Read the model definition and answer for the solid it produces. Units are mm, in the model's axes. A direction names the side the tool comes from. Give positions to 0.01 mm unless a question says otherwise; leave off trailing zeros. Loops run counter-clockwise (first coordinate to the right, second up) from the corner with the lowest first, then second, coordinate; pieces in that order, holes last.
(1) Find section B-B, the plane x = -7.5. Write down the section's boundary in (y, z).
(2) Each of these flat-tipped pins is pushed along its axis until it touches: P1, Ø2, axis at x = -6, z = 5, coming from the -Y side; P2, Ø1.5, axis at x = -4, y = 0, coming from the +Z side; P3, Ø0.6, axis at x = 3.5, z = 5, coming from the +Y side. Where does it stop, or does it pass through?
(3) Determine the mould class of faces 3 (the face through (-16.339, -7.547, 2.958)), 4 (the face through (-2.483, -7.657, 5.246)), 5 (the face through (-2, -8, 5.5)), 6 (the face through (0, 11, 6)) for opening direction X: pulls with the +X half, pulls with the -X half, needs draft (parallel to the pull), parting line crosses it, or undercut.
(4) Straight lines are drawn through the part: probe 1 along X at (y, z) = (-11, 5.25); probe 2 along Z at (x, y) = (-5.5, -5); probe 3 along Z at (x, y) = (4.5, -5.5). For each, find the intervals that lie inside material, in ascending order.
(5) Find section A-A, the plane z = 2.5. Write down the section's boundary in (x, y).
(6) Find section D-D, the plane x = -14. Write down the section's boundary in (y, z), then the cut area to 3 significant figures.
(7) Which of the six approach directions +Z, -Z, +X, -X, +Y, -Y give full straight-line access (tool end or side, diameter ignored) to faces 1 (the face through (0, 6, 0)), 2 (the face through (2.28, -7.66, 5.25))?
(8) Find section C-C, the plane y = 3. Write down the section's boundary in (x, z), then the cut area to 3 significant figures.
```python
from build123d import *

# Parameters (mm, degrees)
F3_DEPTH       = 6
F4_DEPTH       = 5
F7_W           = 8.8009524625
F7_H           = 6.8124858662
F8_DEPTH       = 5.5
F9_DEPTH       = 6
F10_R          = 1.5
F11_DEPTH      = 22.0605344206
F11_DEPTH_BACK = 22.0605344206


with BuildPart() as f3:
    # F2 (on Top) → F3 (new body)
    with BuildSketch(Plane.XY):
        with BuildLine():
            Line((0, 21.6666666667), (0, 25))
            ThreePointArc((0, 25), (-8.7261968456, 24.2326465733), (-17.1845506091, 21.9541395445))
            ThreePointArc((-17.1845506091, 21.9541395445), (-17.6945480382, 17.1258595599), (-22.0595344206, 15))
            ThreePointArc((-22.0595344206, 15), (-16.1790775021, -7.8397846906), (0, -25))
            Line((0, -25), (0, -20.9973518952))
            ThreePointArc((0, -20.9973518952), (-13.1176654632, -6.4864713134), (-18.6418781092, 12.2784394807))
            ThreePointArc((-18.6418781092, 12.2784394807), (-14.9610674668, 15.2181844096), (-13.460154741, 19.6833527404))
            ThreePointArc((-13.460154741, 19.6833527404), (-6.8027439277, 21.1681757581), (0, 21.6666666667))
        make_face()
    extrude(amount=F3_DEPTH)

    # F2 (on Top) → F4 (join)
    with BuildSketch(Plane.XY):
        with BuildLine():
            Line((0, -20.9973518952), (0, 21.6666666667))
            ThreePointArc((0, 21.6666666667), (-6.8027439277, 21.1681757581), (-13.460154741, 19.6833527404))
            ThreePointArc((-13.460154741, 19.6833527404), (-14.9610674668, 15.2181844096), (-18.6418781092, 12.2784394807))
            ThreePointArc((-18.6418781092, 12.2784394807), (-13.1176654632, -6.4864713134), (0, -20.9973518952))
        make_face()
    extrude(amount=F4_DEPTH)

    # F5: F3 across plane


with BuildPart() as f3_1:
    add(f3.part)
    add(f3.part.mirror(Plane.YZ))

    # F7 (on Top) → F8 (join)
    with BuildSketch(Plane.XY):
        with BuildLine():
            Line((5.5992295966, 16.5245700628), (5.5992295966, 13.8685129642))
            Line((5.5992295966, 13.8685129642), (5.5992295966, 7.4030795346))
            Line((5.5992295966, 7.4030795346), (5.5992295966, 1.9538915054))
            Line((5.5992295966, 1.9538915054), (-5.5992295966, 1.9538915054))
            Line((-5.5992295966, 1.9538915054), (-5.5992295966, 7.4030795346))
            Line((-5.5992295966, 7.4030795346), (-5.5992295966, 13.8685129642))
            Line((-5.5992295966, 13.8685129642), (-5.5992295966, 16.5245700628))
            ThreePointArc((-5.5992295966, 16.5245700628), (-12.9710057836, 5.0063042214), (-5.9278514236, -6.7157906769))
            Line((-5.9278514236, -6.7157906769), (-5.9278514236, -19.3214993029))
            Line((-5.9278514236, -19.3214993029), (0, -23.4193839133))
            Line((0, -23.4193839133), (5.9278514236, -20.1235420135))
            Line((5.9278514236, -20.1235420135), (5.9278514236, -6.7157906769))
            ThreePointArc((5.9278514236, -6.7157906769), (12.9710057836, 5.0063042214), (5.5992295966, 16.5245700628))
        make_face()
        with Locations((0.6785687292, -7.6357298531)):
            Rectangle(F7_W, F7_H, mode=Mode.SUBTRACT)
        Polygon((-1.7386174295, -4.9604633823), (-3.247810062, -10.4308445007), (-1.7631669762, -10.4308445007), (-0.2539743437, -4.9604633823), align=None)
        Polygon((0.6177854048, -10.4308445007), (2.1269780373, -4.9604633823), (0.6423349514, -4.9604633823), (-0.8668576811, -10.4308445007), align=None)
        Polygon((2.9987377857, -10.4308445007), (4.5079304183, -4.9604633823), (3.0232873324, -4.9604633823), (1.5140946999, -10.4308445007), align=None)
    extrude(amount=F8_DEPTH)

    # F7 (on Top) → F9 (join)
    with BuildSketch(Plane.XY):
        Polygon((5.5992295966, 7.4030795346), (5.5992295966, 13.8685129642), (0, 17.1012296791), (-5.5992295966, 13.8685129642), (-5.5992295966, 7.4030795346), (0, 4.1703628198), align=None)
    extrude(amount=F9_DEPTH)

    # F10 (on Right) → F11 (cut, two sides)
    with BuildSketch(Plane.YZ) as f11_sk:
        with Locations((9.1423522681, 2.5)):
            Circle(F10_R)
    extrude(amount=-F11_DEPTH, mode=Mode.SUBTRACT)
    extrude(f11_sk.sketch, amount=F11_DEPTH_BACK, mode=Mode.SUBTRACT)


solid = f3_1.part
```
Entries:
1. outline: (-19.14, 0) - (24.43, 0) - (24.43, 6) - (21.06, 6) - (21.06, 5) - (15.41, 5) - (15.41, 5.5) - (-5.76, 5.5) - (-5.76, 5) - (-14.34, 5) - (-14.34, 6) - (-19.14, 6) - close; hole circle Ø3 at (9.14, 2.5)
2. P1: stops at y = -21.37
2. P2: stops at z = 5.5
2. P3: stops at y = 24.9
3. face 3: pulls with the -X half
3. face 4: undercut
3. face 5: undercut
3. face 6: needs draft
4. probe 1: x = -14.27 to -10.21, -5.93 to -3.72, 5.08 to 5.93, 10.21 to 14.27
4. probe 2: z = 0 to 5.5
4. probe 3: z = 0 to 5
5. outline: (-22.06, 15) arc R47.3 ccw to (-21.86, 10.64) - (21.86, 10.64) arc R47.3 ccw to (22.06, 15) arc R5.01 cw to (17.18, 21.95) arc R50 ccw to (-17.18, 21.95) arc R5.01 cw to start; (-21.48, 7.64) arc R47.3 ccw to (0, -25) arc R47.3 ccw to (21.48, 7.64) - close
6. outline: (-11.41, 0) - (23, 0) - (23, 6) - (17.03, 6) - (17.03, 5) - (-4.83, 5) - (-4.83, 6) - (-11.41, 6) - close; hole circle Ø3 at (9.14, 2.5)
6. area: 178 mm2
7. face 1: -Z, +X, -X, +Y, -Y
7. face 2: +Z
8. outline: (-20.51, 0) - (20.51, 0) - (20.51, 6) - (17.06, 6) - (17.06, 5) - (12.84, 5) - (12.84, 5.5) - (5.6, 5.5) - (5.6, 5) - (-5.6, 5) - (-5.6, 5.5) - (-12.84, 5.5) - (-12.84, 5) - (-17.06, 5) - (-17.06, 6) - (-20.51, 6) - close
8. area: 219 mm2
